Can you work these out from the model? Positions are in its coordinate system, mm. Round coordinates to 2 decimals unless told otherwise and drop trailing zeros. Loops run counter-clockwise (first coordinate to the right, second up) from the corner with the lowest first, then second, coordinate; pieces in that order, holes last.
(1) I want a section at B-B on x = 0. Give the number of separate pieces and of enclosed holes in the cut face, plus the area to 3 significant figures.
(2) I want a section at A-A on z = 21. Write out the boundary of the cut face in (x, y).
(3) I want a section at D-D on z = 89. Write out the boundary of the cut face in (x, y).
(4) Will these pins go through, and if not, where does the flat tip stop? pin 1 Ø2.5 at (x, y) = (-14, -1) entering from -Z; pin 2 Ø4.5 at (y, z) = (-1, 44) entering from -X; pin 3 Ø1 at (x, y) = (-12.5, -2) entering from +Z.
(5) If I drill on line 1 along X through (y, z) = (-1.25, 17); line 2 along Z through (x, y) = (-11.5, 2.5); line 3 along Y through (x, z) = (20.5, 136.5), over which ranges is the centre line in solid material (lowest first)?
from build123d import *
from build123d import SkipClean  # not in build123d's __all__

# Parameters (mm, degrees)
F0_R        = 2
F1_DEPTH    = 5
F0_W        = 22
F0_H        = 2
F0_W_2      = 2
F0_H_2      = 6
F0_W_3      = 4
F2_DEPTH    = 4
F3_SIZE     = 5
F4_T1_DEPTH = 219.7493718553
F4_T3_DEPTH = 109.7493718553


# Not quite as in the source:
# - a fillet or chamfer that OpenCascade refuses, or shapes differently, is made with other operations: its cross-section is extruded or revolved along the edge and cut away or added
# - a feature names something its author has since deleted; it is built from what else it names


with BuildPart() as f1:
    # F0 (on Front) → F1 (new body)
    with BuildSketch(Plane.XZ):
        with BuildLine():
            Line((-30, 150), (-30, 80))
            Line((-30, 80), (-2, 80))
            ThreePointArc((-2, 80), (0, 82), (2, 80))
            Line((2, 80), (30, 80))
            Line((30, 80), (30, 150))
            Line((30, 150), (-30, 150))
        make_face()
        with Locations((0, 130)):
            Circle(F0_R, mode=Mode.SUBTRACT)
        with BuildLine():
            Line((-30, 0), (0, 0))
            Line((0, 0), (30, 0))
            Line((30, 0), (30, 80))
            Line((30, 80), (2, 80))
            ThreePointArc((2, 80), (0, 78), (-2, 80))
            Line((-2, 80), (-30, 80))
            Line((-30, 80), (-30, 0))
        make_face()
        Polygon((-11, 24), (-11, 16), (-11, 10), (-11, 8), (-13, 8), (-17, 8), (-19, 8), (-19, 10), (-19, 16), (-19, 24), align=None, mode=Mode.SUBTRACT)
        Polygon((19, 24), (19, 16), (19, 10), (19, 8), (17, 8), (13, 8), (11, 8), (11, 10), (11, 16), (11, 24), align=None, mode=Mode.SUBTRACT)
        Polygon((-19, 54), (-11, 54), (11, 54), (19, 54), (19, 46), (19, 40), (19, 38), (17, 38), (13, 38), (11, 38), (-11, 38), (-13, 38), (-17, 38), (-19, 38), (-19, 40), (-19, 46), (-19, 48), align=None, mode=Mode.SUBTRACT)
        Polygon((30, 0), (0, 0), (-30, 0), (-30, -20), (30, -20), align=None)
    extrude(amount=-F1_DEPTH)

    # F0 (on Front) → F2 (join)
    with BuildSketch(Plane.XZ):
        with BuildLine():
            Line((-30, 0), (0, 0))
            Line((0, 0), (30, 0))
            Line((30, 0), (30, 80))
            Line((30, 80), (2, 80))
            ThreePointArc((2, 80), (0, 78), (-2, 80))
            Line((-2, 80), (-30, 80))
            Line((-30, 80), (-30, 0))
        make_face()
        Polygon((-11, 24), (-11, 16), (-11, 10), (-11, 8), (-13, 8), (-17, 8), (-19, 8), (-19, 10), (-19, 16), (-19, 24), align=None, mode=Mode.SUBTRACT)
        Polygon((19, 24), (19, 16), (19, 10), (19, 8), (17, 8), (13, 8), (11, 8), (11, 10), (11, 16), (11, 24), align=None, mode=Mode.SUBTRACT)
        Polygon((-19, 54), (-11, 54), (11, 54), (19, 54), (19, 46), (19, 40), (19, 38), (17, 38), (13, 38), (11, 38), (-11, 38), (-13, 38), (-17, 38), (-19, 38), (-19, 40), (-19, 46), (-19, 48), align=None, mode=Mode.SUBTRACT)
        with BuildLine():
            Line((-30, 150), (-30, 80))
            Line((-30, 80), (-2, 80))
            ThreePointArc((-2, 80), (0, 82), (2, 80))
            Line((2, 80), (30, 80))
            Line((30, 80), (30, 150))
            Line((30, 150), (-30, 150))
        make_face()
        with Locations((0, 130)):
            Circle(F0_R, mode=Mode.SUBTRACT)
        Polygon((30, 0), (0, 0), (-30, 0), (-30, -20), (30, -20), align=None)
        with Locations((0, 39)):
            Rectangle(F0_W, F0_H)
        with Locations((-18, 43)):
            Rectangle(F0_W_2, F0_H_2)
        with Locations((18, 43)):
            Rectangle(F0_W_2, F0_H_2)
        with Locations((-18, 13)):
            Rectangle(F0_W_2, F0_H_2)
        with Locations((-12, 13)):
            Rectangle(F0_W_2, F0_H_2)
        with Locations((12, 13)):
            Rectangle(F0_W_2, F0_H_2)
        with Locations((18, 13)):
            Rectangle(F0_W_2, F0_H_2)
        with Locations((-15, 39)):
            Rectangle(F0_W_3, F0_H)
        with Locations((15, 39)):
            Rectangle(F0_W_3, F0_H)
        with Locations((-15, 9)):
            Rectangle(F0_W_3, F0_H)
        with Locations((15, 9)):
            Rectangle(F0_W_3, F0_H)
        with Locations((-18, 39)):
            Rectangle(F0_W_2, F0_H)
        with Locations((-12, 39)):
            Rectangle(F0_W_2, F0_H)
        with Locations((12, 39)):
            Rectangle(F0_W_2, F0_H)
        with Locations((18, 39)):
            Rectangle(F0_W_2, F0_H)
        with Locations((-18, 9)):
            Rectangle(F0_W_2, F0_H)
        with Locations((-12, 9)):
            Rectangle(F0_W_2, F0_H)
        with Locations((12, 9)):
            Rectangle(F0_W_2, F0_H)
        with Locations((18, 9)):
            Rectangle(F0_W_2, F0_H)
    with SkipClean():  # cleaning this boolean's faces spoils the solid; the shape is the same uncleaned
        extrude(amount=F2_DEPTH)

    # F3
    f3_edges = [f1.edges().sort_by_distance(p)[0] for p in [
        (-2, -4, 130),
        (2, -4, 80),
    ]]
    chamfer(f3_edges, length=F3_SIZE)

    # F4: fillet of radius 10 on 4 edges, made by hand

    # F4_s2 → F4_t1 (cut)
    with BuildSketch(Plane.XY.offset(-44.8746859277)):
        with BuildLine():
            ThreePointArc((-20.0501256289, -4), (-26.7583295614, -1.4161984871), (-30, 5))
            Line((-30, 5), (-30, -4))
            Line((-30, -4), (-20.0501256289, -4))
        make_face()
        with BuildLine():
            ThreePointArc((20.0501256289, -4), (26.7583295614, -1.4161984871), (30, 5))
            Line((30, 5), (30, -4))
            Line((30, -4), (20.0501256289, -4))
        make_face()
    extrude(amount=F4_T1_DEPTH, mode=Mode.SUBTRACT)

    # F4_s4 → F4_t3 (cut)
    with BuildSketch(Plane.YZ.offset(-54.8746859277)):
        with BuildLine():
            ThreePointArc((-4, 140.0501256289), (-1.4161984871, 146.7583295614), (5, 150))
            Line((5, 150), (-4, 150))
            Line((-4, 150), (-4, 140.0501256289))
        make_face()
        with BuildLine():
            ThreePointArc((-4, -10.0501256289), (-1.4161984871, -16.7583295614), (5, -20))
            Line((5, -20), (-4, -20))
            Line((-4, -20), (-4, -10.0501256289))
        make_face()
    extrude(amount=F4_T3_DEPTH, mode=Mode.SUBTRACT)


solid = f1.part
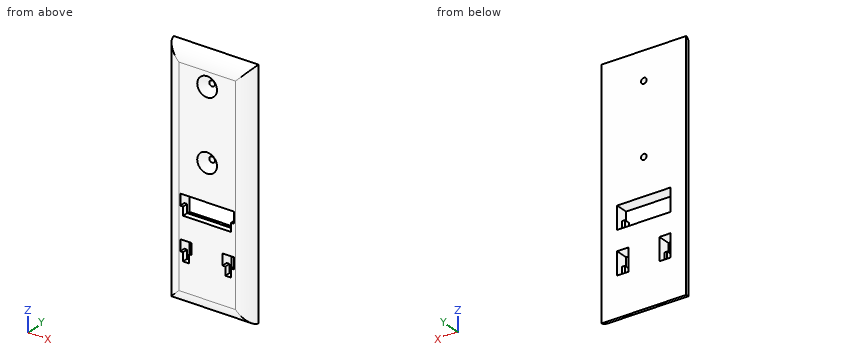
Filled sheet:
1. separate pieces: 4
1. enclosed holes: 0
1. area: 1,230 mm2
2. outline: (-30, 5) arc R10 ccw to (-20.05, -4) - (-19, -4) - (-19, 5) - close; (-11, -4) - (11, -4) - (11, 5) - (-11, 5) - close; (19, -4) - (20.05, -4) arc R10 ccw to (30, 5) - (19, 5) - close
3. outline: (-30, 5) arc R10 ccw to (-20.05, -4) - (20.05, -4) arc R10 ccw to (30, 5) - close
4. pin 1: stops at z = -18.23
4. pin 2: stops at x = -28.85
4. pin 3: stops at z = 146.66
5. line 1: x = -26.94 to -19, -11 to 11, 19 to 26.94
5. line 2: z = -19.42 to 8, 24 to 38, 54 to 149.42
5. line 3: y = -3.99 to 5
